from build123d import *

# Parameters (mm, degrees)
F1_DEPTH = 25.4
F2_R     = 5.08
F3_R     = 5.08


with BuildPart() as f1:
    # F0 (on Top) → F1 (new body)
    with BuildSketch(Plane.XY):
        with BuildLine():
            Line((-26.3964543073, 45.72), (-13.1982270342, 22.8599997931))
            ThreePointArc((-13.1982270342, 22.8599997931), (-13.1982272083, 38.0999999054), (2.04e-08, 45.72))
            Line((2.04e-08, 45.72), (-26.3964543073, 45.72))
        make_face()
        with BuildLine():
            ThreePointArc((-13.1982270342, 22.8599997931), (-7.6199998966, 17.2817727866), (0, 15.24))
            ThreePointArc((0, 15.24), (7.6200000359, 17.281772867), (13.1982271951, 22.8600000717))
            ThreePointArc((13.1982271951, 22.8600000717), (14.7207096034, 26.5355977926), (15.24, 30.48))
            ThreePointArc((15.24, 30.48), (10.7763073525, 41.2563073381), (2.04e-08, 45.72))
            ThreePointArc((2.04e-08, 45.72), (-13.1982272083, 38.0999999054), (-13.1982270342, 22.8599997931))
        make_face()
        with BuildLine():
            ThreePointArc((11.0109, 30.48), (7.785882057, 22.694117943), (0, 19.4691))
            ThreePointArc((0, 19.4691), (-7.785882057, 38.265882057), (11.0109, 30.48))
        make_face(mode=Mode.SUBTRACT)
        with BuildLine():
            ThreePointArc((15.24, 30.48), (14.7207096034, 26.5355977926), (13.1982271951, 22.8600000717))
            Line((13.1982271951, 22.8600000717), (26.3964543073, 45.72))
            Line((26.3964543073, 45.72), (2.04e-08, 45.72))
            ThreePointArc((2.04e-08, 45.72), (10.7763073525, 41.2563073381), (15.24, 30.48))
        make_face()
        with BuildLine():
            ThreePointArc((0, 15.24), (3.9444022474, 14.7207095926), (7.62, 13.1982271537))
            Line((7.62, 13.1982271537), (13.1982271951, 22.8600000717))
            ThreePointArc((13.1982271951, 22.8600000717), (7.6200000359, 17.281772867), (0, 15.24))
        make_face()
        with BuildLine():
            ThreePointArc((-7.62, 13.1982271537), (-3.9444022474, 14.7207095926), (0, 15.24))
            ThreePointArc((0, 15.24), (-7.6199998966, 17.2817727866), (-13.1982270342, 22.8599997931))
            Line((-13.1982270342, 22.8599997931), (-7.62, 13.1982271537))
        make_face()
        with BuildLine():
            ThreePointArc((-5.50545, 9.5357191185), (-2.8498306237, 10.6357126807), (0, 11.0109))
            Line((0, 11.0109), (0, 15.24))
            ThreePointArc((0, 15.24), (-3.9444022474, 14.7207095926), (-7.62, 13.1982271537))
            Line((-7.62, 13.1982271537), (-5.50545, 9.5357191185))
        make_face()
        with BuildLine():
            ThreePointArc((0, 11.0109), (2.8498306237, 10.6357126807), (5.50545, 9.5357191185))
            Line((5.50545, 9.5357191185), (7.62, 13.1982271537))
            ThreePointArc((7.62, 13.1982271537), (3.9444022474, 14.7207095926), (0, 15.24))
            Line((0, 15.24), (0, 11.0109))
        make_face()
        with BuildLine():
            ThreePointArc((-5.5776126233, -9.4936903381), (-11.0108208297, 0.0417548278), (-5.50545, 9.5357191185))
            Line((-5.50545, 9.5357191185), (-7.62, 13.1982271537))
            ThreePointArc((-7.62, 13.1982271537), (-15.2399698636, 0.030307715), (-7.6724341256, -13.1678151031))
            Line((-7.6724341256, -13.1678151031), (-5.5776126233, -9.4936903381))
        make_face()
        with BuildLine():
            Line((0, -15.24), (0, -11.0109))
            ThreePointArc((0, -11.0109), (-2.8901421995, -10.6248292634), (-5.5776126233, -9.4936903381))
            Line((-5.5776126233, -9.4936903381), (-7.6724341256, -13.1678151031))
            ThreePointArc((-7.6724341256, -13.1678151031), (-3.9736694521, -14.7128362692), (0, -15.24))
        make_face()
        with BuildLine():
            Line((7.5678329537, -13.2282086612), (5.4333591334, -9.5769790298))
            ThreePointArc((5.4333591334, -9.5769790298), (2.8096939701, -10.6463861758), (0, -11.0109))
            Line((0, -11.0109), (0, -15.24))
            ThreePointArc((0, -15.24), (3.9153352349, -14.7284673337), (7.5678329537, -13.2282086612))
        make_face()
        with BuildLine():
            ThreePointArc((5.50545, 9.5357191185), (9.5357191185, 5.50545), (11.0109, 0))
            ThreePointArc((11.0109, 0), (9.5148855193, -5.5413782008), (5.4333591334, -9.5769790298))
            Line((5.4333591334, -9.5769790298), (7.5678329537, -13.2282086612))
            ThreePointArc((7.5678329537, -13.2282086612), (13.1831592233, -7.6460390329), (15.24, 0))
            ThreePointArc((15.24, 0), (13.1982271537, 7.62), (7.62, 13.1982271537))
            Line((7.62, 13.1982271537), (5.50545, 9.5357191185))
        make_face()
        with BuildLine():
            ThreePointArc((13.1567863006, -22.7886688902), (7.5842505855, -17.2611973668), (0, -15.24))
            ThreePointArc((0, -15.24), (-7.6556936027, -17.302445012), (-13.2392812888, -22.9315544013))
            ThreePointArc((-13.2392812888, -22.9315544013), (-13.1567861593, -38.1713313515), (0.0824955225, -45.7197767204))
            ThreePointArc((0.0824955225, -45.7197767204), (10.8054345531, -41.2271011961), (15.24, -30.48))
            ThreePointArc((15.24, -30.48), (14.7099800003, -26.4957700381), (13.1567863006, -22.7886688902))
        make_face()
        with BuildLine():
            ThreePointArc((11.0109, -30.48), (-7.785882057, -38.265882057), (0, -19.4691))
            ThreePointArc((0, -19.4691), (7.785882057, -22.694117943), (11.0109, -30.48))
        make_face(mode=Mode.SUBTRACT)
        with BuildLine():
            ThreePointArc((-13.2392812888, -22.9315544013), (-7.6556936027, -17.302445012), (0, -15.24))
            ThreePointArc((0, -15.24), (-3.9736694521, -14.7128362692), (-7.6724341256, -13.1678151031))
            Line((-7.6724341256, -13.1678151031), (-13.2392812888, -22.9315544013))
        make_face()
        with BuildLine():
            Line((13.1567863006, -22.7886688902), (7.5678329537, -13.2282086612))
            ThreePointArc((7.5678329537, -13.2282086612), (3.9153352349, -14.7284673337), (0, -15.24))
            ThreePointArc((0, -15.24), (7.5842505855, -17.2611973668), (13.1567863006, -22.7886688902))
        make_face()
        with BuildLine():
            Line((26.4785625289, -45.5768912828), (13.1567863006, -22.7886688902))
            ThreePointArc((13.1567863006, -22.7886688902), (14.7099800003, -26.4957700381), (15.24, -30.48))
            ThreePointArc((15.24, -30.48), (10.8054345531, -41.2271011961), (0.0824955225, -45.7197767204))
            Line((0.0824955225, -45.7197767204), (26.4785625289, -45.5768912828))
        make_face()
        with BuildLine():
            ThreePointArc((0.0824955225, -45.7197767204), (-13.1567861593, -38.1713313515), (-13.2392812888, -22.9315544013))
            Line((-13.2392812888, -22.9315544013), (-26.3135726335, -45.8626621643))
            Line((-26.3135726335, -45.8626621643), (0.0824955225, -45.7197767204))
        make_face()
    extrude(amount=F1_DEPTH)

    # F2
    f2_edges = [f1.edges().sort_by_distance(p)[0] for p in [
        (26.396454, 45.72, 12.7),
        (26.478563, -45.576891, 12.7),
        (-26.313573, -45.862662, 12.7),
    ]]
    fillet(f2_edges, radius=F2_R)

    # F3
    f3_edges = [f1.edges().sort_by_distance(p)[0] for p in [
        (-26.396454, 45.72, 12.7),
    ]]
    fillet(f3_edges, radius=F3_R)


solid = f1.part
Geometry check sheet. Reference: the model listing, model coordinates, mm. A direction names the side the tool comes from. Give positions to 0.01 mm unless a question says otherwise; leave off trailing zeros. Write each loop counter-clockwise with the first axis right and the second up, starting at its lowest first coordinate (ties: lowest second). Pieces come first, ordered by that corner, then holes.
1) Release check for a two-part mould opening along Y. For faces 1 (the face through (5, 11, 0)), 2 (the face through (22.03, 43.12, 12.88)), 3 (the face through (0, 45.72, 13)) record: released by +Y, released by -Y, zero draft, split by the parting line, or undercut.
Values follow:
face 1: zero draft
face 2: undercut
face 3: released by +Y
2) Cross-section at D-D (y = -15.5). Record the boundary of the cut face in (x, z).
Values follow:
outline: (-9, 0) - (8.9, 0) - (8.9, 25.4) - (-9, 25.4) - close
3) Set-up check for faces 4 (the face through (-14.909, 25.823, 12.522)), 5 (the face through (5, 11, 25.4)): record each of +Z, -Z, +X, -X, +Y, -Y from which the full face is reachable in a straight line by a thin tool's end or side.
Values follow:
face 4: +Z, -Z, -X
face 5: +Z, +X, -X, +Y, -Y
4) Go/stop test with flat-tipped pins: pin 1 Ø4 at (x, y) = (6.5, 5) entering from +Z; pin 2 Ø8 at (y, z) = (-8, 3.5) entering from -X; pin 3 Ø1.5 at (y, z) = (26, 7.5) entering from -X; pin 4 Ø4 at (y, z) = (-32.5, 4) entering from +X. Record where each tip stops, or that it passes through.
Values follow:
pin 1: passes through
pin 2: stops at x = -14.71
pin 3: stops at x = -15.44
pin 4: stops at x = 20
5) Cross-section at B-B (y = -2.5). Record the boundary of the cut face in (x, z).
Values follow:
outline: (-15.03, 0) - (-10.72, 0) - (-10.72, 25.4) - (-15.03, 25.4) - close; (10.72, 0) - (15.03, 0) - (15.03, 25.4) - (10.72, 25.4) - close
6) Cross-section at C-C (y = 40.5). Record the boundary of the cut face in (x, z).
Values follow:
outline: (-22.68, 0) - (-4.57, 0) - (-4.57, 25.4) - (-22.68, 25.4) - close; (4.57, 0) - (22.68, 0) - (22.68, 25.4) - (4.57, 25.4) - close
7) Thickness scan on line 1 (Y direction, x = 2.5, z = 18); line 2 (Y direction, x = -5, z = 21.25); line 3 (X direction, y = 0.5, z = 9.5). Record the ranges inside material, lowest first.
Values follow:
line 1: y = -45.71 to -41.2, -19.76 to -10.72, 10.72 to 19.76, 41.2 to 45.72
line 2: y = -45.75 to -40.29, -20.67 to -9.81, 9.81 to 20.67, 40.29 to 45.72
line 3: x = -15.23 to -11, 11 to 15.23
8) Cross-section at A-A (z = 19.25). Record the boundary of the cut face in (x, y), plus the area to 3 significant figures.
Values follow:
outline: (-22, 38.1) - (-7.62, 13.2) arc R15.24 ccw to (-7.67, -13.17) - (-21.96, -38.22) arc R5.08 ccw to (-17.51, -45.82) - (17.68, -45.62) arc R5.08 ccw to (22.04, -37.98) - (7.57, -13.23) arc R15.24 ccw to (7.62, 13.2) - (22, 38.1) arc R5.08 ccw to (17.6, 45.72) - (-17.6, 45.72) arc R5.08 ccw to start; hole circle Ø22.02 at (0, -30.48); hole circle Ø22.02 at (0, 0); hole circle Ø22.02 at (0, 30.48)
area: 1,690 mm2
